Answer from the drawing. Dimensions are ordinates in mm from the lowest x, y and z of the part. Coordinates: 2 decimals unless noted, no trailing zeros. Write each loop counter-clockwise with the first axis right and the second up, starting at its lowest first coordinate (ties: lowest second). Pieces come first, ordered by that corner, then holes.
1) The part is cut by section A-A (z = 2.5). Give the number of separate pieces and of enclosed holes in the cut face, then the cut area to 3 significant figures.
2) Each of these flat-tipped pins is pushed along its axis until it touches: pin 1 Ø6 at (x, z) = (69, 3.5) entering from -Y; pin 2 Ø3 at (y, z) = (20.5, 15) entering from +X; pin 3 Ø3 at (x, z) = (135, 4) entering from +Y. Where does it stop, or does it pass through?
3) The part is cut by section B-B (y = 18). Determine the outline of the cut face in (x, z), then the cut area to 3 significant figures.
4) Find the intervals of material crossed by line 1 (X direction, y = 12.25, z = 4.25) (1 decimal); line 2 (X direction, y = 22.75, z = 10.25) (1 decimal); line 3 (Z direction, x = 136, y = 15), in increasing order.
5) The part is cut by section C-C (x = 73). Determine the outline of the cut face in (y, z).
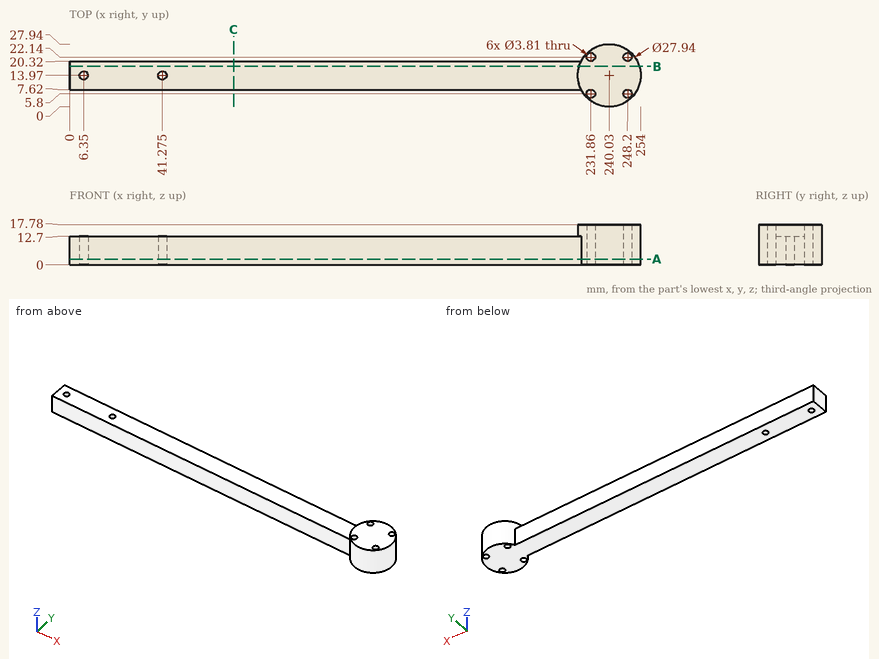
Reported:
1. separate pieces: 1
1. enclosed holes: 6
1. area: 3,420 mm2
2. pin 1: stops at y = 7.62
2. pin 2: stops at x = 253.06
2. pin 3: stops at y = 20.32
3. outline: (0, 0) - (253.41, 0) - (253.41, 17.78) - (226.65, 17.78) - (226.65, 12.7) - (0, 12.7) - close
3. area: 3,350 mm2
4. line 1: x = 0 to 5.5, 7.2 to 40.5, 42.1 to 253.9
4. line 2: x = 229.2 to 230.1, 233.7 to 246.4, 250 to 250.9
4. line 3: z = 0 to 12.7
5. outline: (7.62, 0) - (20.32, 0) - (20.32, 12.7) - (7.62, 12.7) - close
